Part model, mm, in its own coordinate system. Give positions to 0.01 mm unless a question says otherwise; leave off trailing zeros. Write each loop counter-clockwise with the first axis right and the second up, starting at its lowest first coordinate (ties: lowest second). Pieces come first, ordered by that corner, then holes.
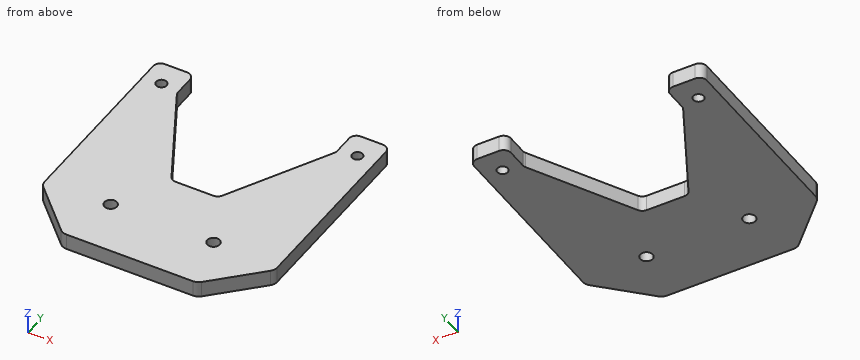
from build123d import *

# Parameters (mm, degrees)
SKETCH1_R           = 2.55
SKETCH1_R_2         = 2.15
BOSS_EXTRUDE1_DEPTH = 6.5
FILLET1_R           = 3
CHAMFER1_SIZE       = 20
FILLET2_R           = 4


with BuildPart() as part:
    # Sketch1 → Boss-Extrude1 (new body)
    with BuildSketch(Plane.XY):
        Polygon((-32.5, 43), (-32.5, 55), (-47.5, 55), (-47.5, -45), (47.5, -45), (47.5, 55), (32.5, 55), (32.5, 43), (9.5, 0), (-9.5, 0), align=None)
        with Locations((-21, -22.5)):
            Circle(SKETCH1_R, mode=Mode.SUBTRACT)
        with Locations((21, -22.5)):
            Circle(SKETCH1_R, mode=Mode.SUBTRACT)
        with Locations((-40, 45)):
            Circle(SKETCH1_R_2, mode=Mode.SUBTRACT)
        with Locations((40, 45)):
            Circle(SKETCH1_R_2, mode=Mode.SUBTRACT)
    extrude(amount=BOSS_EXTRUDE1_DEPTH)

    # Fillet1
    fillet1_edges = [part.edges().sort_by_distance(p)[0] for p in [
        (9.5, 0, 3.25),
        (32.5, 43, 3.25),
        (32.5, 55, 3.25),
        (47.5, 55, 3.25),
        (-47.5, 55, 3.25),
        (-32.5, 55, 3.25),
        (-32.5, 43, 3.25),
        (-9.5, 0, 3.25),
    ]]
    fillet(fillet1_edges, radius=FILLET1_R)

    # Chamfer1
    chamfer1_edges = [part.edges().sort_by_distance(p)[0] for p in [
        (47.5, -45, 3.25),
        (-47.5, -45, 3.25),
    ]]
    chamfer(chamfer1_edges, length=CHAMFER1_SIZE)

    # Fillet2
    fillet2_edges = [part.edges().sort_by_distance(p)[0] for p in [
        (47.5, -25, 3.25),
        (-27.5, -45, 3.25),
        (27.5, -45, 3.25),
        (-47.5, -25, 3.25),
    ]]
    fillet(fillet2_edges, radius=FILLET2_R)


solid = part.part
1) Flat gauge pins, fed straight in: P1, Ø4.5, axis at x = 21, y = -22.5, coming from the +Z side; P2, Ø2, axis at x = 1.5, z = 4, coming from the +Y side; P3, Ø2, axis at x = 29, z = 5, coming from the -Y side. Where does each tip first touch, or does it go through?
Check result:
P1: passes through
P2: stops at y = 0
P3: stops at y = -44.37
2) Saw through at A-A (y = 45). Write the cut outline in (x, z).
Check result:
outline: (-47.5, 0) - (-42.15, 0) - (-42.15, 6.5) - (-47.5, 6.5) - close; (-37.85, 0) - (-32.5, 0) - (-32.5, 6.5) - (-37.85, 6.5) - close; (32.5, 0) - (37.85, 0) - (37.85, 6.5) - (32.5, 6.5) - close; (42.15, 0) - (47.5, 0) - (47.5, 6.5) - (42.15, 6.5) - close
3) Saw through at D-D (y = 29). Write the cut outline in (x, z), and give its area (3 significant figures).
Check result:
outline: (-47.5, 0) - (-25.01, 0) - (-25.01, 6.5) - (-47.5, 6.5) - close; (25.01, 0) - (47.5, 0) - (47.5, 6.5) - (25.01, 6.5) - close
area: 292 mm2
4) Saw through at B-B (x = 21). Write the cut outline in (y, z), and give its area (3 significant figures).
Check result:
outline: (-45, 0) - (-25.05, 0) - (-25.05, 6.5) - (-45, 6.5) - close; (-19.95, 0) - (21.5, 0) - (21.5, 6.5) - (-19.95, 6.5) - close
area: 399 mm2
5) Drill centre lines: L1, parallel to X at y = -23, z = 4.25; L2, parallel to X at y = 45.5, z = 5.5; L3, parallel to X at y = 50, z = 1. Where is each one in solid material? Low to high.
Check result:
L1: x = -47.5 to -23.5, -18.5 to 18.5, 23.5 to 47.5
L2: x = -47.5 to -42.09, -37.91 to -32.5, 32.5 to 37.91, 42.09 to 47.5
L3: x = -47.5 to -32.5, 32.5 to 47.5
6) Saw through at C-C (z = 5). Write the cut outline in (x, y), and give its area (3 significant figures).
Check result:
outline: (-47.5, -23.34) arc R4 ccw to (-46.33, -26.17) - (-28.67, -43.83) arc R4 ccw to (-25.84, -45) - (25.84, -45) arc R4 ccw to (28.67, -43.83) - (46.33, -26.17) arc R4 ccw to (47.5, -23.34) - (47.5, 52) arc R3 ccw to (44.5, 55) - (35.5, 55) arc R3 ccw to (32.5, 52) - (32.5, 43.75) arc R3 cw to (32.15, 42.34) - (10.35, 1.59) arc R3 cw to (7.7, 0) - (-7.7, 0) arc R3 cw to (-10.35, 1.59) - (-32.15, 42.34) arc R3 cw to (-32.5, 43.75) - (-32.5, 52) arc R3 ccw to (-35.5, 55) - (-44.5, 55) arc R3 ccw to (-47.5, 52) - close; hole circle Ø4.3 at (-40, 45); hole circle Ø5.1 at (-21, -22.5); hole circle Ø5.1 at (21, -22.5); hole circle Ø4.3 at (40, 45)
area: 6,440 mm2
